from build123d import *

# Parameters (mm, degrees)
SKETCH015_R     = 7.62
PAD005_DEPTH    = 15.24
POCKET010_DEPTH = 12.7
SKETCH017_R     = 2.54
POCKET011_DEPTH = 15.241


with BuildPart() as part:
    # Sketch015 → Pad005 (new body)
    with BuildSketch(Plane.XY):
        Circle(SKETCH015_R)
    extrude(amount=PAD005_DEPTH)

    # Sketch016 (on DatumPlane) → Pocket010 (cut)
    with BuildSketch(Plane.XY.offset(13.97)):
        with BuildLine():
            ThreePointArc((-1.265583, 7.514167), (0, 6.35), (1.265583, 7.514167))
            ThreePointArc((1.265583, 7.514167), (0, 7.62), (-1.265583, 7.514167))
        make_face()
        with BuildLine():
            ThreePointArc((7.514167, 1.265583), (6.35, 0), (7.514167, -1.265583))
            ThreePointArc((7.514167, -1.265583), (7.62, 0), (7.514167, 1.265583))
        make_face()
        with BuildLine():
            ThreePointArc((1.265583, -7.514167), (0, -6.35), (-1.265583, -7.514167))
            ThreePointArc((-1.265583, -7.514167), (0, -7.62), (1.265583, -7.514167))
        make_face()
        with BuildLine():
            ThreePointArc((-7.514167, -1.265583), (-6.35, 0), (-7.514167, 1.265583))
            ThreePointArc((-7.514167, 1.265583), (-7.62, 0), (-7.514167, -1.265583))
        make_face()
        with BuildLine():
            ThreePointArc((-6.20822, 4.418416), (-4.490128, 4.490128), (-4.418416, 6.20822))
            ThreePointArc((-4.418416, 6.20822), (-5.388154, 5.388154), (-6.20822, 4.418416))
        make_face()
        with BuildLine():
            ThreePointArc((4.418416, 6.20822), (4.490128, 4.490128), (6.20822, 4.418416))
            ThreePointArc((6.20822, 4.418416), (5.388154, 5.388154), (4.418416, 6.20822))
        make_face()
        with BuildLine():
            ThreePointArc((6.20822, -4.418416), (4.490128, -4.490128), (4.418416, -6.20822))
            ThreePointArc((4.418416, -6.20822), (5.388154, -5.388154), (6.20822, -4.418416))
        make_face()
        with BuildLine():
            ThreePointArc((-4.418416, -6.20822), (-4.490128, -4.490128), (-6.20822, -4.418416))
            ThreePointArc((-6.20822, -4.418416), (-5.388154, -5.388154), (-4.418416, -6.20822))
        make_face()
    extrude(amount=-POCKET010_DEPTH, mode=Mode.SUBTRACT)

    # Sketch017 (on Face6 of Pocket010) → Pocket011 (cut, through all)
    with BuildSketch(Plane.XY.offset(15.24)):
        Circle(SKETCH017_R)
    extrude(amount=-POCKET011_DEPTH, mode=Mode.SUBTRACT)


solid = part.part
CAD build for the part. Positions are in the model's coordinates, mm. A direction names the side the tool comes from. Give positions to 0.01 mm unless a question says otherwise; leave off trailing zeros. Write each loop counter-clockwise with the first axis right and the second up, starting at its lowest first coordinate (ties: lowest second). Pieces come first, ordered by that corner, then holes. Notation, with made-up numbers: (32.5, 61) - (89.5, 61) arc R22 ccw to (89.5, 96) - close; hole circle Ø2 at (74.5, 39). An arc over 180 degrees is marked (long way). Answer as CSV lines item,"result".
Q1. Band-saw the part on C-C (z = 1.75). Give the cut face in (x, y).
Result set:
outline,"(-7.51, -1.27) arc R7.62 ccw to (-6.21, -4.42) arc R1.27 cw to (-4.42, -6.21) arc R7.62 ccw to (-1.27, -7.51) arc R1.27 cw to (1.27, -7.51) arc R7.62 ccw to (4.42, -6.21) arc R1.27 cw to (6.21, -4.42) arc R7.62 ccw to (7.51, -1.27) arc R1.27 cw to (7.51, 1.27) arc R7.62 ccw to (6.21, 4.42) arc R1.27 cw to (4.42, 6.21) arc R7.62 ccw to (1.27, 7.51) arc R1.27 cw to (-1.27, 7.51) arc R7.62 ccw to (-4.42, 6.21) arc R1.27 cw to (-6.21, 4.42) arc R7.62 ccw to (-7.51, 1.27) arc R1.27 cw to start; hole circle Ø5.08 at (0, 0)"
Q2. Pull direction Y, two halves, no side cores. Call faces 1 (the face through (-2, 2, 0)), 2 (the face through (0.03, -6.35, 7.71)), 3 (the face through (-0.33, 2.52, 7.73)): released by +Y, released by -Y, zero draft, split by the parting line, or undercut.
Result set:
face 1,"zero draft"
face 2,"released by -Y"
face 3,"undercut"
Q3. Band-saw the part on A-A (x = 0). Give the cut face in (y, z).
Result set:
outline,"(-7.62, 0) - (-2.54, 0) - (-2.54, 15.24) - (-7.62, 15.24) - (-7.62, 13.97) - (-6.35, 13.97) - (-6.35, 1.27) - (-7.62, 1.27) - close; (2.54, 0) - (7.62, 0) - (7.62, 1.27) - (6.35, 1.27) - (6.35, 13.97) - (7.62, 13.97) - (7.62, 15.24) - (2.54, 15.24) - close"
Q4. Flat gauge pins, fed straight in: pin 1 Ø1 at (x, z) = (-2, 4.5) entering from -Y; pin 2 Ø1.5 at (x, z) = (5.5, 11) entering from -Y; pin 3 Ø4 at (y, z) = (-5, 6) entering from -X. Where does each tip first touch, or does it go through?
Result set:
pin 1,"y = -7.47"
pin 2,"y = -4.42"
pin 3,"x = -7"
Q5. Drill centre lines: line 1 (Y direction, x = -5.5, z = 5.5); line 2 (X direction, y = 2, z = 12.75); line 3 (Z direction, x = 4.5, y = 5). Where is each one in solid material? Low to high. Write a range as from..to.
Result set:
line 1,"-4.12..4.12"
line 2,"-7.35..-1.57, 1.57..7.35"
line 3,"0..1.27, 13.97..15.24"
Q6. 3-axis set-ups, long thin cutter, end or side, ignore diameter. For faces 4 (the face through (7, 0, 13.97)), 5 (the face through (-6.35, -0.03, 7.71)), 6 (the face through (0, -7, 13.97)), 7 (the face through (0, 7, 1.27)), 8 (the face through (4.47, 4.51, 7.71)): which of +Z, -Z, +X, -X, +Y, -Y reach the whole face in a straight line?
Result set:
face 4,"+X"
face 5,"-X"
face 6,"-Y"
face 7,"+Y"
face 8,"none"
Q7. Band-saw the part on D-D (x = 2). Give the cut face in (y, z).
Result set:
outline,"(-7.35, 0) - (-1.57, 0) - (-1.57, 15.24) - (-7.35, 15.24) - close; (1.57, 0) - (7.35, 0) - (7.35, 15.24) - (1.57, 15.24) - close"
